Part model, mm, in its own coordinate system. A direction names the side the tool comes from. Round coordinates to 2 decimals unless told otherwise and drop trailing zeros. Loops run counter-clockwise (first coordinate to the right, second up) from the corner with the lowest first, then second, coordinate; pieces in that order, holes last. Notation, with made-up numbers: (88, -7.5) - (134, -7.5) arc R24 cw to (134, 9.5) - close; hole circle Ø5 at (-19.75, -22.5). An arc over 180 degrees is marked (long way). Write each question's results on one line, items separated by ' | '. Start each with the question number.
(1) Mould opens along Y. For faces 4 (the face through (149.225, 1, -127)), 5 (the face through (85.574, -67.202, 1.565)) say: released by +Y, released by -Y, zero draft, split by the parting line, or undercut.
(2) Cut at B-B, the plane y = 32.5. List the corners of the cut face in (x, z) (3 decimals), then the cut area to 3 significant figures.
(3) Tool access for faces 1 (the face through (-2, 1, 0)), 2 (the face through (-2, 1, 3.175)), 3 (the face through (-97.497, 66.677, 1.565)): list every direction of +Z, -Z, +X, -X, +Y, -Y with a clear straight run to the whole face (end or side of a thin tool).
(4) Flat gauge pin, fed straight in: P1, Ø10, axis at x = -91.44, y = 64.77, coming from the +Z side. Where does the tip first touch, or does it go through?
(5) Cut at A-A, the plane x = 119. List the corners of the cut face in (y, z) (3 decimals).
(6) Cut at C-C, the plane x = -91.44. List the corners of the cut face in (y, z) (3 decimals).
(7) Drill centre lines: L1, parallel to Y at x = -91.44, z = 1.6; L2, parallel to X at y = 64, z = 2; L3, parallel to X at y = -51, z = -236.5 (3 decimals). Where is each one in solid material? Low to high.
(8) Cut at D-D, the plane z = -167. List the corners of the cut face in (x, y) (3 decimals).
from build123d import *

# Parameters (mm, degrees)
F0_W     = 304.8
F0_H     = 152.4
F1_DEPTH = 3.175
F4_D     = 12.7
F5_W     = 3.175
F5_H     = 152.4
F6_DEPTH = 257.81
F7_W     = 304.8
F7_H     = 152.4
F8_DEPTH = 3.175


# Not quite as in the source:
# - a length typed as a fraction of an inch, garbled in the dataset ("3 / 203.2 mm" for 3/8 in), is restored


with BuildPart() as f1:
    # F0 (on Top) → F1 (new body)
    with BuildSketch(Plane.XY):
        Rectangle(F0_W, F0_H)
    extrude(amount=F1_DEPTH)

    # F4 (through all)
    with Locations(Plane.XY.offset(3.175)):
        with Locations((-91.44, 64.77), (-91.44, -64.77), (91.44, -64.77), (91.44, 64.77)):
            Hole(F4_D / 2)

    # F5 (on face) → F6 (join)
    with BuildSketch(Plane(origin=(0, 0, 0), x_dir=(1, 0, 0), z_dir=(0, 0, -1))):
        with Locations((-150.8125, 0)):
            Rectangle(F5_W, F5_H)
        with Locations((150.8125, 0)):
            Rectangle(F5_W, F5_H)
    extrude(amount=F6_DEPTH)

    # F7 (on face) → F8 (join)
    with BuildSketch(Plane(origin=(0, 0, -257.81), x_dir=(1, 0, 0), z_dir=(0, 0, -1))):
        Rectangle(F7_W, F7_H)
    extrude(amount=F8_DEPTH)


solid = f1.part
A:
1) face 4: zero draft | face 5: undercut
2) outline: (-152.4, -260.985) - (152.4, -260.985) - (152.4, 3.175) - (-152.4, 3.175) - close; hole (-149.225, -257.81) - (149.225, -257.81) - (149.225, 0) - (-149.225, 0) - close | area: 3,570 mm2
3) face 1: +Y, -Y | face 2: +Z, +X, -X, +Y, -Y | face 3: +Z
4) P1: z = -257.81
5) outline: (-76.2, -260.985) - (76.2, -260.985) - (76.2, -257.81) - (-76.2, -257.81) - close; (-76.2, 0) - (76.2, 0) - (76.2, 3.175) - (-76.2, 3.175) - close
6) outline: (-76.2, -260.985) - (76.2, -260.985) - (76.2, -257.81) - (-76.2, -257.81) - close; (-76.2, 0) - (-71.12, 0) - (-71.12, 3.175) - (-76.2, 3.175) - close; (-58.42, 0) - (58.42, 0) - (58.42, 3.175) - (-58.42, 3.175) - close; (71.12, 0) - (76.2, 0) - (76.2, 3.175) - (71.12, 3.175) - close
7) L1: -76.2 to -71.12, -58.42 to 58.42, 71.12 to 76.2 | L2: -152.4 to -97.74, -85.14 to 85.14, 97.74 to 152.4 | L3: -152.4 to -149.225, 149.225 to 152.4
8) outline: (-152.4, -76.2) - (-149.225, -76.2) - (-149.225, 76.2) - (-152.4, 76.2) - close; (149.225, -76.2) - (152.4, -76.2) - (152.4, 76.2) - (149.225, 76.2) - close
